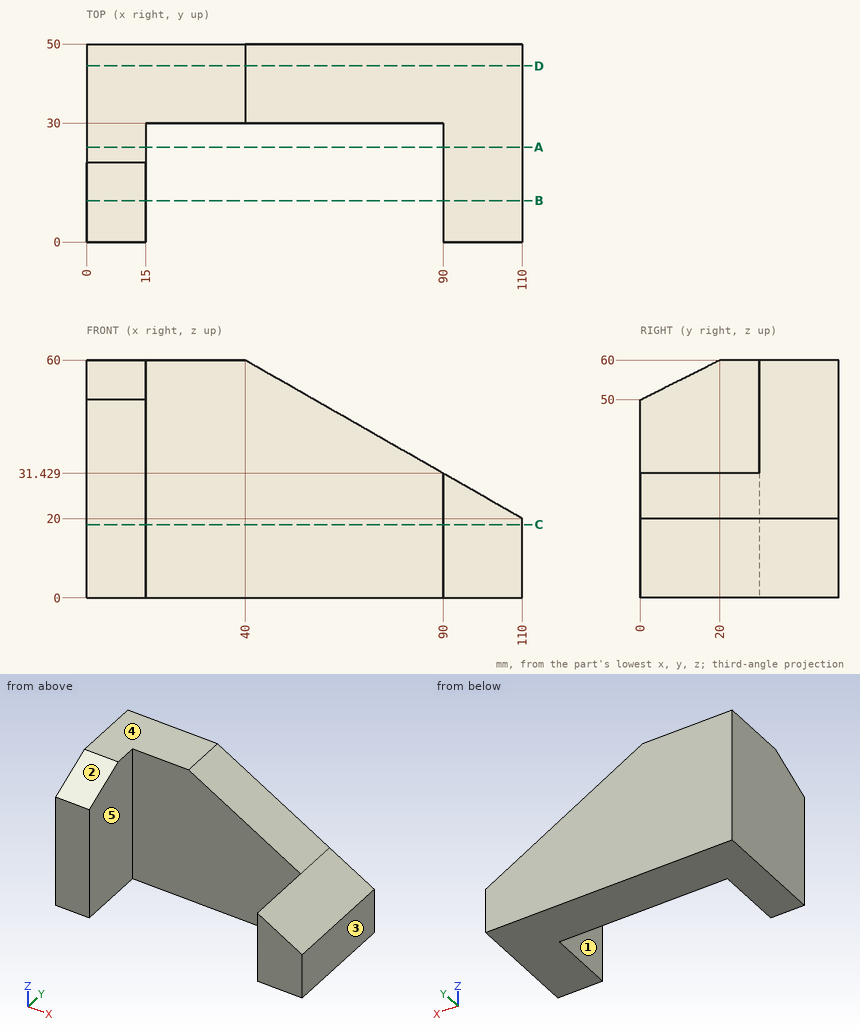
Here's the drawing with two shaded views (mm, measured from the low corner). I have some questions. A direction names the side the tool comes from. Coordinates: 2 decimals unless noted, no trailing zeros. Order: outer loops, then holes, each group sorted by start corner. A loop starts at its lowest first (then second) coordinate and runs counter-clockwise, first axis right, second up.
Q1. Suppose I cut it at A-A on y = 24. Please give me the cut outline in (x, z).
Q2. Which directions (+Z, -Z, +X, -X, +Y, -Y) give clear straight access to the entire face, cutting with the end or side of a thin tool? Please do the marked faces 1 and 2.
Q3. Thinking about a two-plate mould opening in X: for the marked faces 3, 4 and 5, which applies, released by +X, released by -X, zero draft, split by the parting line, or undercut?
Q4. Suppose I cut it at B-B on y = 10.5. Please give me the cut outline in (x, z).
Q5. Suppose I cut it at D-D on y = 44.5. Please give me the cut outline in (x, z).
Q6. Will these pins go through, and if not, where does the flat tip stop? pin 1 (3 mm diameter, centred on x = 82, z = 25, fed in from -Y); pin 2 (1 mm diameter, centred on x = 96, y = 32.5, fed in from +Z) (1 decimal); pin 3 (15 mm diameter, centred on y = 17.5, z = 30.5, fed in from +X).
Q7. Please list where these lines run through material, in increasing order: L1, parallel to X at y = 2.5, z = 12; L2, parallel to X at y = 5, z = 23; L3, parallel to X at y = 24.5, z = 31.5.
Q8. Suppose I cut it at C-C on z = 18.5. Please give me the cut outline in (x, y), and give its area (3 significant figures).
Answer:
1. outline: (0, 0) - (15, 0) - (15, 60) - (0, 60) - close; (90, 0) - (110, 0) - (110, 20) - (90, 31.43) - close
2. face 1: +Z, -Z, -Y
2. face 2: +Z, +X, -X, -Y
3. face 3: released by +X
3. face 4: zero draft
3. face 5: undercut
4. outline: (0, 0) - (15, 0) - (15, 55.25) - (0, 55.25) - close; (90, 0) - (110, 0) - (110, 20) - (90, 31.43) - close
5. outline: (0, 0) - (110, 0) - (110, 20) - (40, 60) - (0, 60) - close
6. pin 1: stops at y = 30
6. pin 2: stops at z = 28.3
6. pin 3: stops at x = 104.75
7. L1: x = 0 to 15, 90 to 110
7. L2: x = 0 to 15, 90 to 104.75
7. L3: x = 0 to 15
8. outline: (0, 0) - (15, 0) - (15, 30) - (90, 30) - (90, 0) - (110, 0) - (110, 50) - (0, 50) - close
8. area: 3,250 mm2
